from build123d import *

# Parameters (mm, degrees)
SKETCH_1_R               = 40
EXTRUDE_1_DEPTH          = 1
SKETCH_2_R               = 1.55
CUT_EXTRUDE_1_DEPTH      = 1
SKETCH_4_R               = 10
CUT_EXTRUDE_3_DEPTH      = 1
CUT_EXTRUDE_4_DEPTH      = 1
PATTERN_CIRCULAR_2_COUNT = 4


with BuildPart() as part:
    # 草图1 → 凸台-拉伸1 (new body)
    with BuildSketch(Plane.XY):
        Circle(SKETCH_1_R)
    extrude(amount=EXTRUDE_1_DEPTH)

    # 草图2 → 切除-拉伸1 (cut)
    with BuildSketch(Plane.XY.offset(1)):
        with Locations((0, 31.5)):
            Circle(SKETCH_2_R)
        with Locations((-31.5, 0)):
            Circle(SKETCH_2_R)
        with Locations((0, -31.5)):
            Circle(SKETCH_2_R)
        with Locations((31.5, 0)):
            Circle(SKETCH_2_R)
    extrude(amount=-CUT_EXTRUDE_1_DEPTH, mode=Mode.SUBTRACT)

    # 草图4 → 切除-拉伸3 (cut)
    with BuildSketch(Plane.XY.offset(1)):
        Circle(SKETCH_4_R)
    extrude(amount=-CUT_EXTRUDE_3_DEPTH, mode=Mode.SUBTRACT)

    # 草图5 → 切除-拉伸4 (cut)
    with BuildSketch(Plane.XY.offset(1)):
        with BuildLine():
            ThreePointArc((9.576564013, -26.311393382), (19.798989873, -19.798989873), (26.311393382, -9.576564013))
            ThreePointArc((26.311393382, -9.576564013), (23.323030995, -3.168000193), (16.914467174, -6.15636258))
            ThreePointArc((16.914467174, -6.15636258), (12.727922061, -12.727922061), (6.15636258, -16.914467174))
            ThreePointArc((6.15636258, -16.914467174), (3.168000193, -23.323030995), (9.576564013, -26.311393382))
        make_face()
    cut_extrude_4 = extrude(amount=-CUT_EXTRUDE_4_DEPTH, mode=Mode.SUBTRACT)

    # 阵列(圆周)2: 切除-拉伸4 ×4 about axis
    pattern_circular_2_axis = Axis((0, 0, 0), (0, 0, 1))
    for i in range(1, PATTERN_CIRCULAR_2_COUNT):
        add(cut_extrude_4.rotate(pattern_circular_2_axis, i * 360 / PATTERN_CIRCULAR_2_COUNT), mode=Mode.SUBTRACT)


solid = part.part
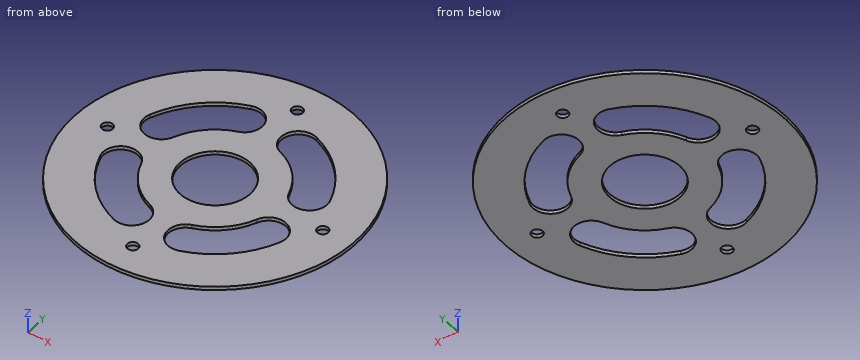
Source: CAD feature listing. Evaluate the final solid. Frame: model axes, mm. Coordinates: 2 decimals unless noted, no trailing zeros. Write each loop counter-clockwise with the first axis right and the second up, starting at its lowest first coordinate (ties: lowest second). Pieces come first, ordered by that corner, then holes. Notation, with made-up numbers: M 51,-0.5 L 94,-0.5 A14 cw 94,16.5 Z; hole C 10,72 d3. An arc over 180 degrees is marked long. Use a Markdown table: item, result.
1) Ray query, L1, parallel to Y at x = 0, z = 0.55; L2, parallel to Y at x = 18.5, z = 0.75; L3, parallel to X at y = 21, z = 0.55. Return the intervals inside material, ascending.
Conclusion:
| item | result |
|---|---|
| L1 | y = -40 to -33.05, -29.95 to -10, 10 to 29.95, 33.05 to 40 |
| L2 | y = -35.46 to -21.02, -3.95 to 3.95, 21.02 to 35.46 |
| L3 | x = -34.04 to -18.52, -2.9 to 2.9, 18.52 to 34.04 |
2) Section A-A, the plane y = 0. Output: boundary loops of the cut face in (x, z).
Conclusion:
| item | result |
|---|---|
| outline | M -40,0 L -33.05,0 L -33.05,1 L -40,1 Z; M -29.95,0 L -10,0 L -10,1 L -29.95,1 Z; M 10,0 L 29.95,0 L 29.95,1 L 10,1 Z; M 33.05,0 L 40,0 L 40,1 L 33.05,1 Z |
3) Section D-D, the plane x = 12. Output: boundary loops of the cut face in (y, z).
Conclusion:
| item | result |
|---|---|
| outline | M -38.16,0 L -25.3,0 L -25.3,1 L -38.16,1 Z; M -13.42,0 L 13.42,0 L 13.42,1 L -13.42,1 Z; M 25.3,0 L 38.16,0 L 38.16,1 L 25.3,1 Z |
4) Section C-C, the plane z = 0.25. Give the number of separate pieces and of enclosed holes in the cut face, then the cut area to 3 significant figures.
Conclusion:
| item | result |
|---|---|
| separate pieces | 1 |
| enclosed holes | 9 |
| area | 3,570 mm^2 |
